Design review of the part shown in the three views and the two pictorial views. Dimensions are in mm from the part's minimum x, y and z. A direction names the side the tool comes from. Coordinates: 2 decimals unless noted, no trailing zeros. Write each loop counter-clockwise with the first axis right and the second up, starting at its lowest first coordinate (ties: lowest second). Pieces come first, ordered by that corner, then holes.
Q1. Take a section at C-C, the plane z = 45. Write out the cut boundary in (x, y).
Q2. For pin 1 Ø1.5 at (x, z) = (27, 8) entering from +Y, flat-tipped, find the tip position at first contact; note if it passes through.
Q3. Take a section at B-B, the plane x = 29. Write out the cut boundary in (y, z), plus the area to 3 significant figures.
Q4. Take a section at A-A, the plane y = 38.5. Write out the cut boundary in (x, z), plus the area to 3 significant figures.
Q5. For the marked faces 5 and 6, list the 3-axis set-ups (+Z, -Z, +X, -X, +Y, -Y) from which the entire face can be reached by the end or side of a thin tool; tool diameter is ignored.
Q6. For L1, parallel to Z at x = 34, y = 39; L2, parallel to Y at x = 22, z = 28.5; L3, parallel to Z at x = 15.5, y = 3, list the stretches that pass through material, from the lowest coordinate up.
Q7. The part is to be moulded in two halves that separate along Z. For the marked faces 1, 2, 3 and 4, say which applies: released by +Z, released by -Z, zero draft, split by the parting line, or undercut.
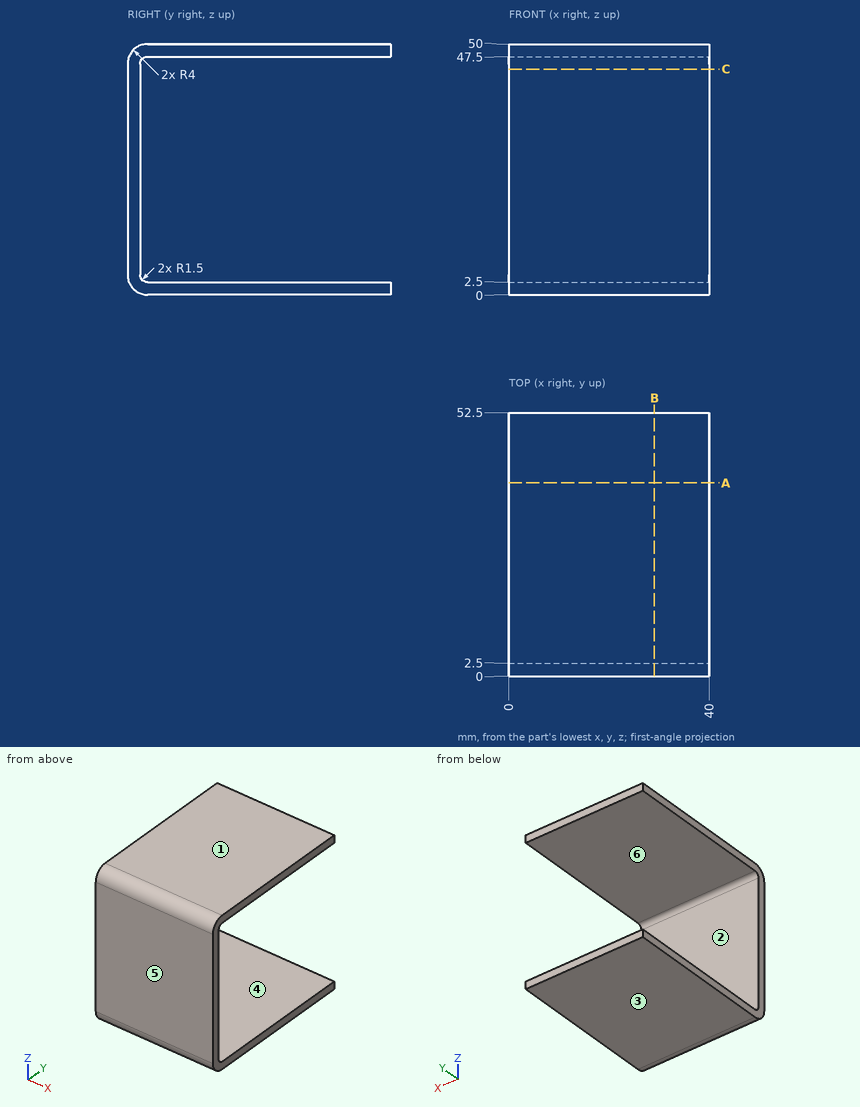
Responses:
1. outline: (0, 0) - (40, 0) - (40, 2.5) - (0, 2.5) - close
2. pin 1: stops at y = 2.5
3. outline: (0, 4) arc R4 ccw to (4, 0) - (52.5, 0) - (52.5, 2.5) - (4, 2.5) arc R1.5 cw to (2.5, 4) - (2.5, 46) arc R1.5 cw to (4, 47.5) - (52.5, 47.5) - (52.5, 50) - (4, 50) arc R4 ccw to (0, 46) - close
3. area: 369 mm2
4. outline: (0, 0) - (40, 0) - (40, 2.5) - (0, 2.5) - close; (0, 47.5) - (40, 47.5) - (40, 50) - (0, 50) - close
4. area: 200 mm2
5. face 5: +Z, -Z, +X, -X, -Y
5. face 6: +X, -X, +Y
6. L1: z = 0 to 2.5, 47.5 to 50
6. L2: y = 0 to 2.5
6. L3: z = 0.13 to 2.88, 47.12 to 49.87
7. face 1: released by +Z
7. face 2: undercut
7. face 3: released by -Z
7. face 4: undercut
